Input: part model. Units: mm. Frame: model coordinates. A direction names the side the tool comes from. Give positions to 0.01 mm unless a question says otherwise; leave off trailing zeros. Loops run counter-clockwise (first coordinate to the right, second up) from the corner with the lowest first, then second, coordinate; pieces in that order, holes last. Notation, with made-up numbers: (73.25, 31) - (94.25, 31) arc R8 ccw to (94.25, 39) - close; hole circle Ø3 at (63.25, -28.5). An arc over 180 degrees is marked (long way). Answer as a JSON object with one key per item and string values.
from build123d import *

# Parameters (mm, degrees)
F0_W     = 152.4
F0_H     = 203.2
F0_R     = 7.14375
F1_DEPTH = 12.7
F3_W     = 101.6
F3_H     = 203.2
F4_DEPTH = 12.7
F6_DEPTH = 6.35


with BuildPart() as f1:
    # F0 (on Top) → F1 (new body)
    with BuildSketch(Plane.XY):
        Rectangle(F0_W, F0_H)
        with Locations((-50.8, -76.2)):
            Circle(F0_R, mode=Mode.SUBTRACT)
        with Locations((50.8, -76.2)):
            Circle(F0_R, mode=Mode.SUBTRACT)
        with Locations((-50.8, 76.2)):
            Circle(F0_R, mode=Mode.SUBTRACT)
        with Locations((50.8, 76.2)):
            Circle(F0_R, mode=Mode.SUBTRACT)
    extrude(amount=F1_DEPTH)



with BuildPart() as f4:
    # F3 (on offset) → F4 (new body)
    with BuildSketch(Plane(origin=(0, 0, 295.402), x_dir=(1, 0, 0), z_dir=(0, 0, -1))):
        with Locations((-152.4, 0)):
            Rectangle(F3_W, F3_H)
        with BuildLine():
            ThreePointArc((-114.3, -54.737), (-108.712, -60.325), (-114.3, -65.913))
            Line((-114.3, -65.913), (-190.5, -65.913))
            ThreePointArc((-190.5, -65.913), (-196.088, -60.325), (-190.5, -54.737))
            Line((-190.5, -54.737), (-114.3, -54.737))
        make_face(mode=Mode.SUBTRACT)
        with BuildLine():
            Line((-114.3, 54.737), (-190.5, 54.737))
            ThreePointArc((-190.5, 54.737), (-196.088, 60.325), (-190.5, 65.913))
            Line((-190.5, 65.913), (-114.3, 65.913))
            ThreePointArc((-114.3, 65.913), (-108.712, 60.325), (-114.3, 54.737))
        make_face(mode=Mode.SUBTRACT)
    extrude(amount=F4_DEPTH)


with BuildPart() as f1_1:
    add(f1.part)

    add(f4.part)  # F6 merges F4
    # F5 (on face) → F6 (join, symmetric)
    with BuildSketch(Plane(origin=(0, 101.6, 0), x_dir=(-1, 0, 0), z_dir=(0, 1, 0))):
        Polygon((-76.2, 12.7), (76.2, 12.7), (203.2, 282.702), (101.6, 282.702), align=None)
    extrude(amount=F6_DEPTH, both=True)

    # F7: F1 across plane


with BuildPart() as f1_2:
    add(f1_1.part)
    add(f1_1.part.mirror(Plane.XZ))


solid = f1_2.part
Item 1: Cut plane C-C (z = 198.5). Return loops of the section in (x, y).
Geometry check:
{"outline": "(-163.59, -107.95) - (-46.15, -107.95) - (-46.15, -95.25) - (-163.59, -95.25) - close; (-163.59, 95.25) - (-46.15, 95.25) - (-46.15, 107.95) - (-163.59, 107.95) - close"}
Item 2: Cut plane A-A (y = 44). Return loops of the section in (x, z).
Geometry check:
{"outline": "(-203.2, 282.7) - (-101.6, 282.7) - (-101.6, 295.4) - (-203.2, 295.4) - close; (-76.2, 0) - (76.2, 0) - (76.2, 12.7) - (-76.2, 12.7) - close"}
Item 3: Access query for faces 4 (the face through (-1, 101.6, 6)), 5 (the face through (-62, 95.25, 150)), 6 (the face through (-153, 54.737, 289)), 7 (the face through (-1, -101.6, 6)). Directions: +Z, -Z, +X, -X, +Y, -Y. A direction counts if a zero-diameter tool reaches every point of the face in a straight line with its end or side. Return the directions, or none.
Geometry check:
{"face 4": "-Z, +X, -X, +Y", "face 5": "+X, -X", "face 6": "+Z, -Z", "face 7": "-Z, +X, -X, -Y"}
Item 4: Contact query for flat-ended pins moving along their axis: P1, Ø4, axis at x = -162.5, z = 289, coming from the +Y side; P2, Ø5, axis at x = -133.5, y = 106, coming from the +Z side; P3, Ø4, axis at x = -2, z = 9, coming from the -Y side; P4, Ø3, axis at x = -54.5, y = -74, coming from the +Z side. Output: stop coordinate, or through.
Geometry check:
{"P1": "stops at y = 101.6", "P2": "stops at z = 282.7", "P3": "stops at y = -101.6", "P4": "passes through"}
Item 5: Material intervals for line 1 (Y direction, x = 50, z = 3); line 2 (X direction, y = -76, z = 3); line 3 (Y direction, x = -121, z = 187), sorted ascending. Write a range as [from, to].
Geometry check:
{"line 1": "y = [-101.6, -83.3], [-69.1, 69.1], [83.3, 101.6]", "line 2": "x = [-76.2, -57.94], [-43.66, 43.66], [57.94, 76.2]", "line 3": "y = [-107.95, -95.25], [95.25, 107.95]"}
Item 6: Mould query, pull axis X, two halves, no side actions, for faces 1 (the face through (-13.945, -101.689, 149.591)), 2 (the face through (-196.087, 60.448, 289.141)), 3 (the face through (-138.81, 101.69, 145.81)). Classes: released by +X, released by -X, zero draft, split by the parting line, or undercut.
Geometry check:
{"face 1": "released by +X", "face 2": "undercut", "face 3": "released by -X"}
Item 7: Cut plane B-B (y = -76.2). Return loops of the section in (x, z), then the cut area to 3 significant figures.
Geometry check:
{"outline": "(-203.2, 282.7) - (-101.6, 282.7) - (-101.6, 295.4) - (-203.2, 295.4) - close; (-76.2, 0) - (-57.94, 0) - (-57.94, 12.7) - (-76.2, 12.7) - close; (-43.66, 0) - (43.66, 0) - (43.66, 12.7) - (-43.66, 12.7) - close; (57.94, 0) - (76.2, 0) - (76.2, 12.7) - (57.94, 12.7) - close", "area": "2,860 mm2"}
Item 8: Cut plane D-D (x = -164.5). Return loops of the section in (y, z).
Geometry check:
{"outline": "(-107.95, 200.43) - (-95.25, 200.43) - (-95.25, 282.7) - (-65.91, 282.7) - (-65.91, 295.4) - (-101.6, 295.4) - (-101.6, 282.7) - (-107.95, 282.7) - close; (-54.74, 282.7) - (54.74, 282.7) - (54.74, 295.4) - (-54.74, 295.4) - close; (65.91, 282.7) - (95.25, 282.7) - (95.25, 200.43) - (107.95, 200.43) - (107.95, 282.7) - (101.6, 282.7) - (101.6, 295.4) - (65.91, 295.4) - close"}
